Geometry check sheet. Reference: the model listing, model coordinates, mm. A direction names the side the tool comes from. Coordinates: 2 decimals unless noted, no trailing zeros. Loops run counter-clockwise (first coordinate to the right, second up) from the corner with the lowest first, then second, coordinate; pieces in that order, holes last. Notation, with made-up numbers: (65, 41) -> (81, 41) arc R11 cw to (81, 49) -> close; hole circle Ø3 at (7, 48.25). An arc over 180 degrees is marked (long way). Answer as a JSON object with one key per item and string values.
from build123d import *

# Parameters (mm, degrees)
BOSS_EXTRUDE1_DEPTH = 4
SKETCH4_W           = 7
SKETCH4_H           = 20
BOSS_EXTRUDE3_DEPTH = 5
BOSS_EXTRUDE4_DEPTH = 30
SKETCH6_W           = 5
SKETCH6_H           = 5
CUT_EXTRUDE2_DEPTH  = 30
SKETCH7_W           = 5
SKETCH7_H           = 5
BOSS_EXTRUDE5_DEPTH = 2
CHAMFER1_SIZE       = 3


with BuildPart() as part:
    # Sketch1 → Boss-Extrude1 (new body)
    with BuildSketch(Plane(origin=(0, 0, 0), x_dir=(1, 0, 0), z_dir=(0, 1, 0))):
        Polygon((-114, 0), (-86.446344316, 0), (0, 106.160035841), (0, 140), (0, 145), (-20, 145), (-20, 115.438596491), align=None)
    extrude(amount=BOSS_EXTRUDE1_DEPTH)

    # Sketch4 → Boss-Extrude3 (add)
    with BuildSketch(Plane(origin=(0, 4, 0), x_dir=(1, 0, 0), z_dir=(0, 1, 0))):
        with Locations((-3.5, 135)):
            Rectangle(SKETCH4_W, SKETCH4_H)
    extrude(amount=BOSS_EXTRUDE3_DEPTH)

    # Sketch5 → Boss-Extrude4 (add)
    with BuildSketch(Plane(origin=(0, 4, 0), x_dir=(1, 0, 0), z_dir=(0, 1, 0))):
        Polygon((-86.446344316, 0), (-104, 0), (-104, 2), (-109, 2), (-109, 0), (-114, 0), (-109.928571429, 5), (-82.374833619, 5), align=None)
    extrude(amount=BOSS_EXTRUDE4_DEPTH)

    # Sketch6 → Cut-Extrude2 (cut)
    with BuildSketch(Plane.XY.offset(-2)):
        with Locations((-106.5, 6.5)):
            Rectangle(SKETCH6_W, SKETCH6_H)
    extrude(amount=-CUT_EXTRUDE2_DEPTH, mode=Mode.SUBTRACT)

    # Sketch7 → Boss-Extrude5 (add)
    with BuildSketch(Plane.XY.offset(-2)):
        with Locations((-106.5, 31.5)):
            Rectangle(SKETCH7_W, SKETCH7_H)
    extrude(amount=BOSS_EXTRUDE5_DEPTH)

    # Chamfer1
    chamfer1_edges = [part.edges().sort_by_distance(p)[0] for p in [
        (-96.151702524, 34, -5),
    ]]
    chamfer(chamfer1_edges, length=CHAMFER1_SIZE)


solid = part.part
1. Section check A-A, the plane y = 18. Record the boundary of the cut face in (x, z).
Evaluation:
{"outline": "(-114, 0) -> (-109.93, -5) -> (-82.37, -5) -> (-86.45, 0) -> (-104, 0) -> (-104, -2) -> (-109, -2) -> (-109, 0) -> close"}
2. Depth check by flat-ended pin: P1, Ø1.5, axis at y = 16, z = -2, coming from the +X side; P2, Ø5.5, axis at x = -3.5, y = 5.5, coming from the +Z side; P3, Ø4, axis at x = -35.5, z = -74, coming from the +Y side; P4, Ø8, axis at x = -75.5, y = 24.5, coming from the -Z side. Enter the tip coordinate at first touch or a pass-through.
Evaluation:
{"P1": "stops at x = -84.21", "P2": "stops at z = -99.03", "P3": "stops at y = 4", "P4": "passes through"}
3. Thickness scan on probe 1 along Z at (x, y) = (-101, 26.5); probe 2 along Y at (x, z) = (-86.5, -15.5); probe 3 along Z at (x, y) = (-105.5, 25). Record the ranges inside material, lowest first. Write a range as from..to.
Evaluation:
{"probe 1": "z = -5..0", "probe 2": "y = 0..4", "probe 3": "z = -5..-2"}
4. Section check B-B, the plane z = -130. Record the boundary of the cut face in (x, y), then the cut area to 3 significant figures.
Evaluation:
{"outline": "(-20, 0) -> (0, 0) -> (0, 9) -> (-7, 9) -> (-7, 4) -> (-20, 4) -> close", "area": "115 mm^2"}
5. Mould release check, pull along Y, two halves, no side actions. Record for faces 4 (the face through (-98, 32, -4)), 5 (the face through (-45, 0, -67)), 6 (the face through (-109, 14, -1)): released by +Y, released by -Y, zero draft, split by the parting line, or undercut.
Evaluation:
{"face 4": "released by +Y", "face 5": "released by -Y", "face 6": "undercut"}
6. Tool access check on faces 1 (the face through (-7, 6, -135)), 2 (the face through (-107, 9, -3)), 3 (the face through (-20, 2, -130)). Record the directions out of +Z, -Z, +X, -X, +Y, -Y that give a thin tool (end or side, any length) a straight path to the whole face; none if there is none.
Evaluation:
{"face 1": "+Z, -Z, -X, +Y", "face 2": "+Z, -Z", "face 3": "-Z, -X, +Y, -Y"}
7. Section check D-D, the plane z = -48.5. Record the boundary of the cut face in (x, y).
Evaluation:
{"outline": "(-74.51, 0) -> (-46.95, 0) -> (-46.95, 4) -> (-74.51, 4) -> close"}
8. Section check C-C, the plane x = -93.5. Record the boundary of the cut face in (y, z), then the cut area to 3 significant figures.
Evaluation:
{"outline": "(0, -25.18) -> (4, -25.18) -> (4, -5) -> (31, -5) -> (34, -2) -> (34, 0) -> (0, 0) -> close", "area": "246 mm^2"}
